The model under review builds one solid part; all positions refer to its coordinate system, in mm. Face numbers are marked on the shaded views. A direction names the side the tool comes from. Round coordinates to 2 decimals unless told otherwise and drop trailing zeros. Order: outer loops, then holes, each group sorted by start corner. A loop starts at its lowest first (then second) coordinate and runs counter-clockwise, first axis right, second up. Notation, with made-up numbers: (36, -29.5) -> (58, -29.5) arc R7 ccw to (58, -23.5) -> close; hole circle Ø6 at (-13, -16.75). An arc over 180 degrees is marked (long way). Use a Markdown table: item, result. Add a question column.
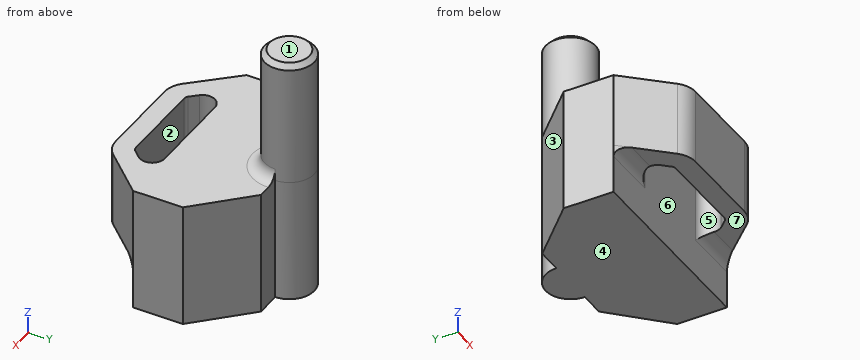
```python
from build123d import *

# Parameters (mm, degrees)
F1_DEPTH     = 5
F2_DEPTH     = 10
F3_SIZE      = 0.2
F5_DEPTH     = 3
F6_T1_DEPTH  = 3
F6_T6_DEPTH  = 2.3418509092
F6_T12_DEPTH = 2.3418509092
F6_T16_ANGLE = 180
F6_T21_DEPTH = 2.3418509092
F6_T25_DEPTH = 5.8592538582
F6_T33_DEPTH = 5.8592538582
F6_T38_DEPTH = 2.3418509092


# Not quite as in the source:
# - a fillet or chamfer that OpenCascade refuses, or shapes differently, is made with other operations: its cross-section is extruded or revolved along the edge and cut away or added


with BuildPart() as f1:
    # F0 (on Top) → F1 (new body)
    with BuildSketch(Plane.XY):
        with BuildLine():
            Line((0, 2), (0, 0))
            Line((0, 0), (8, 0))
            Line((8, 0), (8, 2))
            Line((8, 2), (6, 4))
            Line((6, 4), (5, 4))
            ThreePointArc((5, 4), (4, 3), (3, 4))
            Line((3, 4), (2, 4))
            Line((2, 4), (0, 2))
        make_face()
        with BuildLine():
            ThreePointArc((5, 4), (4, 5), (3, 4))
            Line((3, 4), (5, 4))
        make_face()
        with BuildLine():
            Line((5, 4), (3, 4))
            ThreePointArc((3, 4), (4, 3), (5, 4))
        make_face()
    extrude(amount=F1_DEPTH)

    # F0 (on Top) → F2 (join)
    with BuildSketch(Plane.XY):
        with BuildLine():
            ThreePointArc((5, 4), (4, 5), (3, 4))
            Line((3, 4), (5, 4))
        make_face()
        with BuildLine():
            Line((5, 4), (3, 4))
            ThreePointArc((3, 4), (4, 3), (5, 4))
        make_face()
    extrude(amount=F2_DEPTH)

    # F3
    f3_edges = [f1.edges().sort_by_distance(p)[0] for p in [
        (5, 4, 10),
    ]]
    chamfer(f3_edges, length=F3_SIZE)

    # F4 (on face) → F5 (join)
    with BuildSketch(Plane.XY.offset(5)):
        with BuildLine():
            Line((1.0894362964, 0), (0, 0))
            Line((0, 0), (1.5518551177, -1.6787983581))
            ThreePointArc((1.5518551177, -1.6787983581), (1.8854295116, -1.9161873057), (2.286179834, -2))
            Line((2.286179834, -2), (5.713820166, -2))
            ThreePointArc((5.713820166, -2), (6.1145704884, -1.9161873057), (6.4481448823, -1.6787983581))
            Line((6.4481448823, -1.6787983581), (8, 0))
            Line((8, 0), (6.9105637036, 0))
            Line((6.9105637036, 0), (5.8606851097, -1.1357596721))
            ThreePointArc((5.8606851097, -1.1357596721), (5.7939702307, -1.1832374617), (5.713820166, -1.2000000007))
            Line((5.713820166, -1.2000000007), (2.286179834, -1.2000000007))
            ThreePointArc((2.286179834, -1.2000000007), (2.2060297693, -1.1832374617), (2.1393148903, -1.1357596721))
            Line((2.1393148903, -1.1357596721), (1.0894362964, 0))
        make_face()
    extrude(amount=-F5_DEPTH)

    # F6: fillet of radius 0.5 on 5 edges, made by hand

    # F6_s2 → F6_t1 (join)
    with BuildSketch(Plane.XY.offset(2)):
        with BuildLine():
            ThreePointArc((5.7668622302, 0.0004), (6.2255674394, -0.2996248388), (6.1345147512, -0.8401197793))
            Line((6.1345147512, -0.8401197793), (6.1712800033, -0.8741050071))
            ThreePointArc((6.1712800033, -0.8741050071), (6.5591576145, -0.4539093578), (6.9473289557, -0.0339852278))
            Line((6.9473289557, -0.0339852278), (6.9105637036, 0.0500667501))
            ThreePointArc((6.9105637036, 0.0500667501), (6.3387129669, 0.0500667501), (5.7668622302, 0.0504667501))
            Line((5.7668622302, 0.0504667501), (5.7668622302, 0.0004))
        make_face()
        with BuildLine():
            ThreePointArc((2.2331377698, 0.0004), (1.7744325606, -0.2996248388), (1.8654852488, -0.8401197793))
            Line((1.8654852488, -0.8401197793), (1.8287199967, -0.8741050071))
            ThreePointArc((1.8287199967, -0.8741050071), (1.4408423855, -0.4539093578), (1.0526710443, -0.0339852278))
            Line((1.0526710443, -0.0339852278), (1.0894362964, 0.0500667501))
            ThreePointArc((1.0894362964, 0.0500667501), (1.6612870331, 0.0500667501), (2.2331377698, 0.0504667501))
            Line((2.2331377698, 0.0504667501), (2.2331377698, 0.0004))
        make_face()
    extrude(amount=F6_T1_DEPTH)


with BuildPart() as f6_tool4:
    # F6_s5 → F6_t6 (new body)
    with BuildSketch(Plane.YZ.offset(8)):
        with BuildLine():
            ThreePointArc((0.0004, 1.4990343146), (-0.1464466094, 1.8535533906), (-0.5009656854, 2.0004))
            Line((-0.5009656854, 2.0004), (-0.5009656854, 2.0505365685))
            ThreePointArc((-0.5009656854, 2.0505365685), (-0.2504828427, 2.0501365685), (0, 2.0501365685))
            Line((0, 2.0501365685), (0.0501365685, 2))
            ThreePointArc((0.0501365685, 2), (0.0501365685, 1.7495171573), (0.0505365685, 1.4990343146))
            Line((0.0505365685, 1.4990343146), (0.0004, 1.4990343146))
        make_face()
    extrude(amount=-F6_T6_DEPTH)

    split(bisect_by=Plane(origin=(4.3138623121, -3.9876672942, 0), x_dir=(0, 0, 1), z_dir=(-0.7343247163, 0.6787983581, 0)), keep=Keep.TOP)

    split(bisect_by=Plane(origin=(3.7264025395, -3.4446286081, 0), x_dir=(0, 0, 1), z_dir=(0.7343247163, -0.6787983581, 0)), keep=Keep.TOP)


with BuildPart() as f1_1:
    add(f1.part)

    # F6_t3: union F6_tool4
    add(f6_tool4.part)


with BuildPart() as f6_tool10:
    # F6_s11 → F6_t12 (new body)
    with BuildSketch(Plane.YZ.offset(2.3418509092)):
        with BuildLine():
            ThreePointArc((0.0004, 1.4990343146), (-0.1464466094, 1.8535533906), (-0.5009656854, 2.0004))
            Line((-0.5009656854, 2.0004), (-0.5009656854, 2.0505365685))
            ThreePointArc((-0.5009656854, 2.0505365685), (-0.2504828427, 2.0501365685), (0, 2.0501365685))
            Line((0, 2.0501365685), (0.0501365685, 2))
            ThreePointArc((0.0501365685, 2), (0.0501365685, 1.7495171573), (0.0505365685, 1.4990343146))
            Line((0.0505365685, 1.4990343146), (0.0004, 1.4990343146))
        make_face()
    extrude(amount=-F6_T12_DEPTH)

    split(bisect_by=Plane(origin=(0, 0, 0), x_dir=(0, 0, 1), z_dir=(0.7343247163, 0.6787983581, 0)), keep=Keep.TOP)

    split(bisect_by=Plane(origin=(0.5874597726, 0.543038686, 0), x_dir=(0, 0, 1), z_dir=(-0.7343247163, -0.6787983581, 0)), keep=Keep.TOP)


with BuildPart() as f1_2:
    add(f1_1.part)

    # F6_t9: union F6_tool10
    add(f6_tool10.part)

    # F6_s15 → F6_t16 (revolve)
    with BuildSketch(Plane.XZ.offset(-4)):
        with BuildLine():
            ThreePointArc((4.9996, 5.5009656854), (5.1464466094, 5.1464466094), (5.5009656854, 4.9996))
            Line((5.5009656854, 4.9996), (5.5009656854, 4.9494634315))
            ThreePointArc((5.5009656854, 4.9494634315), (5.2504828427, 4.9498634315), (5, 4.9498634315))
            Line((5, 4.9498634315), (4.9498634315, 5))
            ThreePointArc((4.9498634315, 5), (4.9498634315, 5.2504828427), (4.9494634315, 5.5009656854))
            Line((4.9494634315, 5.5009656854), (4.9996, 5.5009656854))
        make_face()
    revolve(axis=Axis((4, 4, 5), (0, 0, -1)), revolution_arc=F6_T16_ANGLE)


with BuildPart() as f6_tool19:
    # F6_s20 → F6_t21 (new body)
    with BuildSketch(Plane.YZ.offset(8)):
        with BuildLine():
            ThreePointArc((0.0004, 1.4990343146), (-0.1464466094, 1.8535533906), (-0.5009656854, 2.0004))
            Line((-0.5009656854, 2.0004), (-0.5009656854, 2.0505365685))
            ThreePointArc((-0.5009656854, 2.0505365685), (-0.2504828427, 2.0501365685), (0, 2.0501365685))
            Line((0, 2.0501365685), (0.0501365685, 2))
            ThreePointArc((0.0501365685, 2), (0.0501365685, 1.7495171573), (0.0505365685, 1.4990343146))
            Line((0.0505365685, 1.4990343146), (0.0004, 1.4990343146))
        make_face()
    extrude(amount=-F6_T21_DEPTH)

    split(bisect_by=Plane(origin=(3.7264025395, -3.4446286081, 0), x_dir=(0, 0, 1), z_dir=(-0.7343247163, 0.6787983581, 0)), keep=Keep.TOP)


with BuildPart() as f6_tool23:
    # F6_s24 → F6_t25 (new body)
    with BuildSketch(Plane.XY.offset(5)):
        with BuildLine():
            ThreePointArc((5.7668622302, 0.0004), (6.2255674394, -0.2996248388), (6.1345147512, -0.8401197793))
            Line((6.1345147512, -0.8401197793), (6.1712800033, -0.8741050071))
            ThreePointArc((6.1712800033, -0.8741050071), (6.5591576145, -0.4539093578), (6.9473289557, -0.0339852278))
            Line((6.9473289557, -0.0339852278), (6.9105637036, 0.0500667501))
            ThreePointArc((6.9105637036, 0.0500667501), (6.3387129669, 0.0500667501), (5.7668622302, 0.0504667501))
            Line((5.7668622302, 0.0504667501), (5.7668622302, 0.0004))
        make_face()
    extrude(amount=-F6_T25_DEPTH)

    split(bisect_by=Plane.XY, keep=Keep.TOP)

    split(bisect_by=Plane.XY.offset(2), keep=Keep.BOTTOM)


with BuildPart() as f6_tool19_1:
    add(f6_tool19.part)

    # F6_t28: intersect F6_tool23
    add(f6_tool23.part, mode=Mode.INTERSECT)


with BuildPart() as f1_3:
    add(f1_2.part)

    # F6_t17: union F6_tool19
    add(f6_tool19_1.part)


with BuildPart() as f6_tool31:
    # F6_s32 → F6_t33 (new body)
    with BuildSketch(Plane.XY.offset(5)):
        with BuildLine():
            ThreePointArc((2.2331377698, 0.0004), (1.7744325606, -0.2996248388), (1.8654852488, -0.8401197793))
            Line((1.8654852488, -0.8401197793), (1.8287199967, -0.8741050071))
            ThreePointArc((1.8287199967, -0.8741050071), (1.4408423855, -0.4539093578), (1.0526710443, -0.0339852278))
            Line((1.0526710443, -0.0339852278), (1.0894362964, 0.0500667501))
            ThreePointArc((1.0894362964, 0.0500667501), (1.6612870331, 0.0500667501), (2.2331377698, 0.0504667501))
            Line((2.2331377698, 0.0504667501), (2.2331377698, 0.0004))
        make_face()
    extrude(amount=-F6_T33_DEPTH)

    split(bisect_by=Plane.XY, keep=Keep.TOP)

    split(bisect_by=Plane.XY.offset(2), keep=Keep.BOTTOM)


with BuildPart() as f6_tool36:
    # F6_s37 → F6_t38 (new body)
    with BuildSketch(Plane.YZ.offset(2.3418509092)):
        with BuildLine():
            ThreePointArc((0.0004, 1.4990343146), (-0.1464466094, 1.8535533906), (-0.5009656854, 2.0004))
            Line((-0.5009656854, 2.0004), (-0.5009656854, 2.0505365685))
            ThreePointArc((-0.5009656854, 2.0505365685), (-0.2504828427, 2.0501365685), (0, 2.0501365685))
            Line((0, 2.0501365685), (0.0501365685, 2))
            ThreePointArc((0.0501365685, 2), (0.0501365685, 1.7495171573), (0.0505365685, 1.4990343146))
            Line((0.0505365685, 1.4990343146), (0.0004, 1.4990343146))
        make_face()
    extrude(amount=-F6_T38_DEPTH)

    split(bisect_by=Plane(origin=(0.5874597726, 0.543038686, 0), x_dir=(0, 0, 1), z_dir=(0.7343247163, 0.6787983581, 0)), keep=Keep.TOP)


with BuildPart() as f6_tool31_1:
    add(f6_tool31.part)

    # F6_t40: intersect F6_tool36
    add(f6_tool36.part, mode=Mode.INTERSECT)


with BuildPart() as f1_4:
    add(f1_3.part)

    # F6_t29: union F6_tool31
    add(f6_tool31_1.part)


solid = f1_4.part
```
Q1. Add section A-A (x = 4). Write out the cut boundary in (y, z), then the cut area to 3 significant figures.
Q2. Machinability: for the marked faces 4, 5, 6 and 7, which of the approach directions +Z, -Z, +X, -X, +Y, -Y give a long, thin tool a straight path to every point of the face, cutting with its end or side? Answer none if there is none.
Q3. Mouldability with a two-part tool opening along Y and no side actions: class the marked faces 1, 2 and 3 as pulls with the +Y half, pulls with the -Y half, needs draft (parallel to the pull), parting line crosses it, or undercut.
Q4. Insertion check: pin 1 (0.8 mm diameter, centred on x = 2.5, z = 2, fed in from +Y); pin 2 (1 mm diameter, centred on y = -1, z = 4, fed in from +X); pin 3 (1.2 mm diameter, centred on x = 2.5, y = -1.5, fed in from -Z). Each pin has a flat end and moves straight along its axis. Give the tip position at first contact, or say it passes through.
Q5. Wall thickness on line 1 (Z direction, x = 0.5, y = 1.5); line 2 (Y direction, x = 4.25, z = 3.5); line 3 (Z direction, x = 6, y = -1.5): over which ranges is each line inside the solid? List them lowest first. Write a range as [from, to].
Q6. Add section D-D (x = 7). Write out the cut boundary in (y, z), then the cut area to 3 significant figures.
Q7. Add section C-C (y = 0.25). Write out the cut boundary in (x, z).
Q8. Add section B-B (z = 4.75). Write out the cut boundary in (x, y).
Report:
| question | item | result |
|---|---|---|
| 1 | outline | (-2, 2) -> (-1.2, 2) -> (-1.2, 5) -> (-2, 5) -> close; (0, 0) -> (5, 0) -> (5, 9.8) -> (4.8, 10) -> (3.2, 10) -> (3, 9.8) -> (3, 5.48) arc R0.5 cw to (2.52, 5) -> (0, 5) -> close |
| 1 | area | 37.4 mm² |
| 2 | face 4 | -Z, +X, -X, +Y, -Y |
| 2 | face 5 | +Z, -Z |
| 2 | face 6 | -Z |
| 2 | face 7 | -Z, +X, -X, -Y |
| 3 | face 1 | needs draft |
| 3 | face 2 | undercut |
| 3 | face 3 | pulls with the +Y half |
| 4 | pin 1 | stops at y = 4 |
| 4 | pin 2 | stops at x = 7.54 |
| 4 | pin 3 | stops at z = 2 |
| 5 | line 1 | z = [0, 5] |
| 5 | line 2 | y = [-2, -1.2], [0, 4.97] |
| 5 | line 3 | z = [2, 5] |
| 6 | outline | (-1.08, 2) -> (-0.48, 2) arc R0.5 cw to (0, 1.52) -> (0, 0) -> (3, 0) -> (3, 5) -> (-1.08, 5) -> close |
| 6 | area | 18.3 mm² |
| 7 | outline | (0, 0) -> (8, 0) -> (8, 5) -> (0, 5) -> close |
| 8 | outline | (0, 0) -> (1.55, -1.68) arc R1 ccw to (2.29, -2) -> (5.71, -2) arc R1 ccw to (6.45, -1.68) -> (8, 0) -> (8, 2) -> (6, 4) -> (5, 4) arc R1 ccw to (3, 4) -> (2, 4) -> (0, 2) -> close; hole (1.85, -0.83) -> (2.14, -1.14) arc R0.2 ccw to (2.29, -1.2) -> (5.71, -1.2) arc R0.2 ccw to (5.86, -1.14) -> (6.15, -0.83) arc R0.5 ccw to (5.79, 0) -> (2.21, 0) arc R0.5 ccw to start |
